```python
from build123d import *

# Parameters (mm, degrees)
F2_DEPTH = 5.72
F3_DEPTH = 4.56
F4_W     = 2
F4_H     = 0.73
F5_DEPTH = 18.941


with BuildPart() as f2:
    # F1 (on Top) → F2 (new body)
    with BuildSketch(Plane.XY):
        with BuildLine():
            ThreePointArc((0, 3.2), (0.9372583002, 0.9372583002), (3.2, 0))
            Line((3.2, 0), (12.15, 0))
            Line((12.15, 0), (12.15, 1.16))
            Line((12.15, 1.16), (12.15, 10.81))
            Line((12.15, 10.81), (12.15, 19.6))
            ThreePointArc((12.15, 19.6), (12.0035533906, 19.9535533906), (11.65, 20.1))
            Line((11.65, 20.1), (3.2, 20.1))
            ThreePointArc((3.2, 20.1), (0.9372583002, 19.1627416998), (0, 16.9))
            Line((0, 16.9), (0, 3.2))
        make_face()
    extrude(amount=F2_DEPTH)

    # F1 (on Top) → F3 (join)
    with BuildSketch(Plane.XY):
        with BuildLine():
            Line((12.15, 10.81), (12.15, 1.16))
            Line((12.15, 1.16), (31.15, 1.16))
            ThreePointArc((31.15, 1.16), (33.2713203436, 2.0386796564), (34.15, 4.16))
            Line((34.15, 4.16), (34.15, 7.81))
            ThreePointArc((34.15, 7.81), (33.2713203436, 9.9313203436), (31.15, 10.81))
            Line((31.15, 10.81), (12.15, 10.81))
        make_face()
    extrude(amount=F3_DEPTH)

    # F4 (on face) → F5 (cut, through all)
    with BuildSketch(Plane.XZ.offset(-1.16)):
        with Locations((13.15, 0.545)):
            Rectangle(F4_W, F4_H)
        with Locations((16.25, 0.545)):
            Rectangle(F4_W, F4_H)
        with Locations((19.35, 0.545)):
            Rectangle(F4_W, F4_H)
        with Locations((22.45, 0.545)):
            Rectangle(F4_W, F4_H)
        with Locations((25.55, 0.545)):
            Rectangle(F4_W, F4_H)
        with Locations((28.65, 0.545)):
            Rectangle(F4_W, F4_H)
        with Locations((31.75, 0.545)):
            Rectangle(F4_W, F4_H)
    extrude(amount=-F5_DEPTH, mode=Mode.SUBTRACT)


solid = f2.part
```
Model file for the job. Use its own axes, mm. A direction names the side the tool comes from. Coordinates: 2 decimals unless noted, no trailing zeros. Order: outer loops, then holes, each group sorted by start corner. A loop starts at its lowest first (then second) coordinate and runs counter-clockwise, first axis right, second up. Notation, with made-up numbers: (-18.75, -6) - (-11.75, -6) arc R34 ccw to (-11.75, 27) - close; hole circle Ø3 at (-11, -15.75). An arc over 180 degrees is marked (long way). Return JSON: item names as keys, results as strings. Group by question number.
1) Saw through at A-A, the plane x = 23. Write the cut outline in (y, z), plus the area to 3 significant figures.
2) Tool access for faces 1 (the flat face through (22, 1.16, 2)), 2 (the flat face through (8, 0, 3)), 3 (the flat face through (29, 6, 0.18)), 4 (the flat face through (23, 6, 4.56)): list every direction of +Z, -Z, +X, -X, +Y, -Y with a clear straight run to the whole face (end or side of a thin tool).
3) Saw through at C-C, the plane z = 5.3. Write the cut outline in (x, y).
4) Mould opens along X. For faces 5 (the cylindrical face through (33.3, 9.9, 2.2)), 6 (the flat face through (6, 10, 5.72)), 7 (the flat face through (29, 6, 0.91)) say: released by +X, released by -X, zero draft, split by the parting line, or undercut.
5) Saw through at B-B, the plane z = 3.5. Write the cut outline in (x, y), plus the area to 3 significant figures.
6) Flat gauge pins, fed straight in: P1, Ø1.6, axis at x = 32, y = 6, coming from the +Z side; P2, Ø6, axis at x = 21.5, y = 15, coming from the +Z side; P3, Ø3, axis at x = 17, z = 4, coming from the -Y side. Where does each tip first touch, or does it go through?
7) Probe line 1 (Z direction, x = 25.5, y = 2.25); line 2 (Y direction, x = 19, z = 0.95); line 3 (X direction, y = 16.5, z = 5.45). List the from-to ranges inside material, lowest first. Write a range as from..to.
8) Saw through at D-D, the plane x = 18. Write the cut outline in (y, z), plus the area to 3 significant figures.
Values found:
{
 "1": {"outline": "(1.16, 0) - (10.81, 0) - (10.81, 0.18) - (1.16, 0.18) - close; (1.16, 0.91) - (10.81, 0.91) - (10.81, 4.56) - (1.16, 4.56) - close", "area": "37.0 mm²"},
 "2": {"face 1": "+Z, -Z, +X, -Y", "face 2": "+Z, -Z, +X, -X, -Y", "face 3": "+Y, -Y", "face 4": "+Z, +X, +Y, -Y"},
 "3": {"outline": "(0, 3.2) arc R3.2 ccw to (3.2, 0) - (12.15, 0) - (12.15, 19.6) arc R0.5 ccw to (11.65, 20.1) - (3.2, 20.1) arc R3.2 ccw to (0, 16.9) - close"},
 "4": {"face 5": "released by +X", "face 6": "zero draft", "face 7": "undercut"},
 "5": {"outline": "(0, 3.2) arc R3.2 ccw to (3.2, 0) - (12.15, 0) - (12.15, 1.16) - (31.15, 1.16) arc R3 ccw to (34.15, 4.16) - (34.15, 7.81) arc R3 ccw to (31.15, 10.81) - (12.15, 10.81) - (12.15, 19.6) arc R0.5 ccw to (11.65, 20.1) - (3.2, 20.1) arc R3.2 ccw to (0, 16.9) - close", "area": "448 mm²"},
 "6": {"P1": "stops at z = 4.56", "P2": "passes through", "P3": "stops at y = 1.16"},
 "7": {"line 1": "z = 0..0.18, 0.91..4.56", "line 2": "y = 1.16..10.81", "line 3": "x = 0..12.15"},
 "8": {"outline": "(1.16, 0) - (10.81, 0) - (10.81, 4.56) - (1.16, 4.56) - close", "area": "44.0 mm²"}
}
